Autodesk Inventor part; units mm, degrees
ref_plane "YZ Plane" through (0, 0, 0) normal (1, 0, 0) x (0, 1, 0)
ref_plane "XZ Plane" through (0, 0, 0) normal (0, 1, 0) x (-1, 0, 0)
ref_plane "XY Plane" through (0, 0, 0) normal (0, 0, 1) x (1, 0, 0)
sketch "Sketch1" plane through (0, 0, 0) normal (0, 0, 1) x (1, 0, 0)
  line L0 (-17, 37.5) -> (17, 37.5)
  line L1 (17, 37.5) -> (17, -37.5)
  line L2 (17, -37.5) -> (-17, -37.5)
  line L3 (-17, -37.5) -> (-17, 37.5)
  line L4 (-17, 37.5) -> (17, -37.5) construction
  line L5 (17, 37.5) -> (-17, -37.5) construction
  point P0 (0, 0)
  dimension "d0" = 34
  dimension "d1" = 75
extrude "Extrusion1" add sketch "Sketch1" along normal mid plane 77
fillet "Fillet1" radius 7 4 edges at (17, 37.5, 0) (-17, 37.5, 0) (17, -37.5, 0) (-17, -37.5, 0)
sketch "Sketch2" plane through (0, 0, -38.5) normal (0, 0, -1) x (-1, 0, 0)
  circle A0 centre (0, 4.15) radius 4.1
  circle A1 centre (0, -4.15) radius 4.1
  line L0 (0, 0) -> (24.0198, 0) construction
  line L1 (-4.1, 4.15) -> (-4.1, -4.15)
  line L2 (4.1, 4.15) -> (4.1, -4.15)
  dimension "d5" = 8.2
  dimension "d6" = 16.5
extrude "Extrusion2" cut sketch "Sketch2" against normal blind 15
sketch "Sketch3" plane through (0, 0, -23.5) normal (0, 0, -1) x (-1, 0, 0)
  circle A0 centre (0, 4.15) radius 1
  circle A1 centre (0, -4.15) radius 1
  arc A2 (4.1, 4.15) -> (-4.1, 4.15) centre (0, 4.15) ccw
  arc A3 (-4.1, -4.15) -> (4.1, -4.15) centre (0, -4.15) ccw
  point P0 (0, 0)
  dimension "d9" = 2
extrude "Extrusion3" add sketch "Sketch3" along normal blind 15
fillet "Fillet2" radius 1 2 edges at (1, 4.15, -38.5) (1, -4.15, -38.5)
sketch "Sketch4" plane through (0, 0, 38.5) normal (0, 0, 1) x (1, 0, 0)
  line L0 (-6.25, 29.7073) -> (6.25, 29.7073)
  line L1 (6.25, 29.7073) -> (6.25, 24.7073)
  line L2 (6.25, 24.7073) -> (-6.25, 24.7073)
  line L3 (-6.25, 24.7073) -> (-6.25, 29.7073)
  line L4 (-6.25, 29.7073) -> (6.25, 24.7073) construction
  line L5 (6.25, 29.7073) -> (-6.25, 24.7073) construction
  line L6 (-6.25, 19.2073) -> (6.25, 19.2073)
  line L7 (6.25, 19.2073) -> (6.25, 14.2073)
  line L8 (6.25, 14.2073) -> (-6.25, 14.2073)
  line L9 (-6.25, 14.2073) -> (-6.25, 19.2073)
  line L10 (-6.25, 19.2073) -> (6.25, 14.2073) construction
  line L11 (6.25, 19.2073) -> (-6.25, 14.2073) construction
  line L12 (-6.25, 8.7073) -> (6.25, 8.7073)
  line L13 (6.25, 8.7073) -> (6.25, 3.7073)
  line L14 (6.25, 3.7073) -> (-6.25, 3.7073)
  line L15 (-6.25, 3.7073) -> (-6.25, 8.7073)
  line L16 (-6.25, 8.7073) -> (6.25, 3.7073) construction
  line L17 (6.25, 8.7073) -> (-6.25, 3.7073) construction
  line L18 (-4.1, -2.8572) -> (4.1, -2.8572)
  line L19 (4.1, -2.8572) -> (4.1, -5.3572)
  line L20 (4.1, -5.3572) -> (-4.1, -5.3572)
  line L21 (-4.1, -5.3572) -> (-4.1, -2.8572)
  line L22 (-4.1, -2.8572) -> (4.1, -5.3572) construction
  line L23 (4.1, -2.8572) -> (-4.1, -5.3572) construction
  line L24 (-4.1, -14.3572) -> (4.1, -14.3572)
  line L25 (4.1, -14.3572) -> (4.1, -16.8572)
  line L26 (4.1, -16.8572) -> (-4.1, -16.8572)
  line L27 (-4.1, -16.8572) -> (-4.1, -14.3572)
  line L28 (-4.1, -14.3572) -> (4.1, -16.8572) construction
  line L29 (4.1, -14.3572) -> (-4.1, -16.8572) construction
  line L30 (-4.1, -25.8572) -> (4.1, -25.8572)
  line L31 (4.1, -25.8572) -> (4.1, -28.3572)
  line L32 (4.1, -28.3572) -> (-4.1, -28.3572)
  line L33 (-4.1, -28.3572) -> (-4.1, -25.8572)
  line L34 (-4.1, -25.8572) -> (4.1, -28.3572) construction
  line L35 (4.1, -25.8572) -> (-4.1, -28.3572) construction
  point P0 (0, 0)
  point P1 (0, 27.2073)
  point P2 (0, 16.7073)
  point P3 (0, 6.2073)
  point P4 (0, -4.1072)
  point P5 (0, -15.6072)
  point P6 (0, -27.1072)
  dimension "d5" = 8.2
  dimension "d6" = 16.5
  dimension "d14" = 12.5
  dimension "d15" = 5
  dimension "d16" = 5.5
  dimension "d17" = 5.5
  dimension "d18" = 8.2
  dimension "d19" = 2.5
  dimension "d20" = 9
  dimension "d21" = 9
extrude "Extrusion4" cut sketch "Sketch4" against normal blind 10
equation "\"d17\" = d16"
equation "\"d21\" = d20"
properties part number "PowerUSB"
Geometry: final body of the model. Coordinates: model frame, mm. A direction names the side the tool comes from. Give positions to 0.01 mm unless a question says otherwise; leave off trailing zeros. Loops run counter-clockwise (first coordinate to the right, second up) from the corner with the lowest first, then second, coordinate; pieces in that order, holes last. Notation, with made-up numbers: M 53,6 L 85,6 A22 ccw 85,23 Z; hole C 84.5,6 d4. An arc over 180 degrees is marked long. Put each result on its own line as item: value.
1) Cut plane A-A, the plane z = -32.5. Return the cut outline in (x, y).
Computed values:
outline: M -17,-30.5 A7 ccw -10,-37.5 L 10,-37.5 A7 ccw 17,-30.5 L 17,30.5 A7 ccw 10,37.5 L -10,37.5 A7 ccw -17,30.5 Z; C 0,-4.15 d2; C 0,4.15 d2; hole M -4.1,-4.15 A4.1 ccw 4.1,-4.15 L 4.1,4.15 A4.1 ccw -4.1,4.15 Z
2) First-contact query: P1, Ø3, axis at x = 12, z = 1.5, coming from the -Y side. Flat tip, straight axial feed; report the tip coordinate or a pass-through.
Computed values:
P1: stops at y = -37.48
3) Reachability of faces 5 (the flat face through (0, -25.857, 34)), 6 (the flat face through (-17, 0, -1)), 7 (the cylindrical face through (0.217, -3.174, -30.402)) from +Z, -Z, +X, -X, +Y, -Y: full face, straight path, thin tool, end or side. Return the list, or none.
Computed values:
face 5: +Z
face 6: +Z, -Z, -X, +Y, -Y
face 7: -Z
4) Cut plane B-B, the plane z = 23. Return the cut outline in (x, y), plus the area to 3 significant figures.
Computed values:
outline: M -17,-30.5 A7 ccw -10,-37.5 L 10,-37.5 A7 ccw 17,-30.5 L 17,30.5 A7 ccw 10,37.5 L -10,37.5 A7 ccw -17,30.5 Z
area: 2,510 mm^2
5) Material intervals for L1, parallel to X at y = -5, z = -28.5; L2, parallel to Z at x = -1.5, y = 2; L3, parallel to X at y = -32.5, z = 14.5, sorted ascending. Write a range as from..to.
Computed values:
L1: x = -17..-4.01, -0.53..0.53, 4.01..17
L2: z = -23.5..38.5
L3: x = -16.71..16.71
6) Mould query, pull axis X, two halves, no side actions, for faces 1 (the cylindrical face through (-15, -35.4, 0.5)), 2 (the flat face through (-6.25, 6, 34)), 3 (the flat face through (0, 1, 38.5)), 4 (the cylindrical face through (14.9, 35.5, -0.5)). Classes: released by +X, released by -X, zero draft, split by the parting line, or undercut.
Computed values:
face 1: released by -X
face 2: undercut
face 3: zero draft
face 4: released by +X
